```python
from build123d import *

# Parameters (mm, degrees)
F1_DEPTH = 3
F2_W     = 7
F2_H     = 9.4
F3_DEPTH = 3
F4_R     = 1


with BuildPart() as f1:
    # F0 (on Top) → F1 (new body)
    with BuildSketch(Plane.XY):
        with BuildLine():
            ThreePointArc((-2.4, -1.3425721582), (-2.6610618181, -0.6937218463), (-2.75, 0))
            Line((-2.75, 0), (-3.5, 0))
            ThreePointArc((-3.5, 0), (-3.2132538026, -1.3874436926), (-2.4, -2.5475478406))
            Line((-2.4, -2.5475478406), (-2.4, -1.3425721582))
        make_face()
        with BuildLine():
            ThreePointArc((-2.75, 0), (0, 2.75), (2.75, 0))
            Line((2.75, 0), (3.5, 0))
            ThreePointArc((3.5, 0), (0, 3.5), (-3.5, 0))
            Line((-3.5, 0), (-2.75, 0))
        make_face()
        with BuildLine():
            Line((3.5, 0), (2.75, 0))
            ThreePointArc((2.75, 0), (2.6610618181, -0.6937218463), (2.4, -1.3425721582))
            Line((2.4, -1.3425721582), (2.4, -2.5475478406))
            ThreePointArc((2.4, -2.5475478406), (3.2132538026, -1.3874436926), (3.5, 0))
        make_face()
        with BuildLine():
            ThreePointArc((-3.5, 0), (0, 3.5), (3.5, 0))
            Line((3.5, 0), (3.5, 4))
            Line((3.5, 4), (-3.5, 4))
            Line((-3.5, 4), (-3.5, 0))
        make_face()
    extrude(amount=F1_DEPTH)

    # F2 (on face) → F3 (join)
    with BuildSketch(Plane(origin=(0, 4, 0), x_dir=(-1, 0, 0), z_dir=(0, 1, 0))):
        with Locations((0, -1.7)):
            Rectangle(F2_W, F2_H)
    extrude(amount=F3_DEPTH)

    # F4
    f4_edges = [f1.edges().sort_by_distance(p)[0] for p in [
        (0, 7, 3),
        (-2.4, -1.342572, 1.5),
        (2.4, -1.342572, 1.5),
    ]]
    fillet(f4_edges, radius=F4_R)


solid = f1.part
```
For this review, take the finished solid that the model builds, in its own axes (mm). A direction names the side the tool comes from. Coordinates: 2 decimals unless noted, no trailing zeros. Loops run counter-clockwise (first coordinate to the right, second up) from the corner with the lowest first, then second, coordinate; pieces in that order, holes last.
1. Mouldability with a two-part tool opening along X and no side actions: class faces 4 (the cylindrical face through (-0.049, 6.699, 2.715)), 5 (the flat face through (3.5, 4.2, -0.7)), 6 (the flat face through (-2.4, -2, 1)) as +X half, -X half, draft (parallel to the pull), parting line (faces both ways), or undercut.
2. Add section D-D, the plane z = 2.25. Give the boundary of the cut face in (x, y).
3. Add section C-C, the plane y = -0.5. Give the boundary of the cut face in (x, z), then the cut area to 3 significant figures.
4. Insertion check: P1, Ø1.1, axis at y = -2.5, z = 2, coming from the -X side; P2, Ø0.8, axis at y = -2, z = 1, coming from the +X side. Each pin has a flat end and moves straight along its axis. Give the tip position at first contact, or say it passes through.
5. For line 1 (Z direction, x = -3, y = -1); line 2 (Y direction, x = -2.75, z = -1); line 3 (Y direction, x = 2.5, z = 2.25), list the stretches that pass through material, from the lowest coordinate up.
6. Add section B-B, the plane x = 0. Give the boundary of the cut face in (y, z).
7. Add section A-A, the plane z = 0.75. Give the boundary of the cut face in (x, y), then the cut area to 4 significant figures.
8. For faces 1 (the flat face through (2.4, -2, 1)), 2 (the flat face through (0, 3, 0)), 3 (the flat face through (0, 7, -2)), list the 3-axis set-ups (+Z, -Z, +X, -X, +Y, -Y) from which the entire face can be reached by the end or side of a thin tool; tool diameter is ignored.
Result:
1. face 4: draft
1. face 5: +X half
1. face 6: undercut
2. outline: (-3.5, 0) arc R3.5 ccw to (-2.4, -2.55) - (-2.4, -1.58) arc R1 ccw to (-2.49, -1.16) arc R2.75 cw (long way) to (2.49, -1.16) arc R1 ccw to (2.4, -1.58) - (2.4, -2.55) arc R3.5 ccw to (3.5, 0) - (3.5, 6.97) - (-3.5, 6.97) - close
3. outline: (-3.46, 0) - (-2.7, 0) - (-2.7, 3) - (-3.46, 3) - close; (2.7, 0) - (3.46, 0) - (3.46, 3) - (2.7, 3) - close
3. area: 4.56 mm2
4. P1: stops at x = -2.91
4. P2: stops at x = 3.11
5. line 1: z = 0 to 3
5. line 2: y = 4 to 7
5. line 3: y = -2.45 to -1.15, 1.15 to 6.97
6. outline: (2.75, 0) - (4, 0) - (4, -6.4) - (7, -6.4) - (7, 2) arc R1 ccw to (6, 3) - (2.75, 3) - close
7. outline: (-3.5, 0) arc R3.5 ccw to (-2.4, -2.55) - (-2.4, -1.58) arc R1 ccw to (-2.49, -1.16) arc R2.75 cw (long way) to (2.49, -1.16) arc R1 ccw to (2.4, -1.58) - (2.4, -2.55) arc R3.5 ccw to (3.5, 0) - (3.5, 7) - (-3.5, 7) - close
7. area: 40.35 mm2
8. face 1: +Z, -Z, -Y
8. face 2: -Z, +X, -X, -Y
8. face 3: +Z, -Z, +X, -X, +Y
